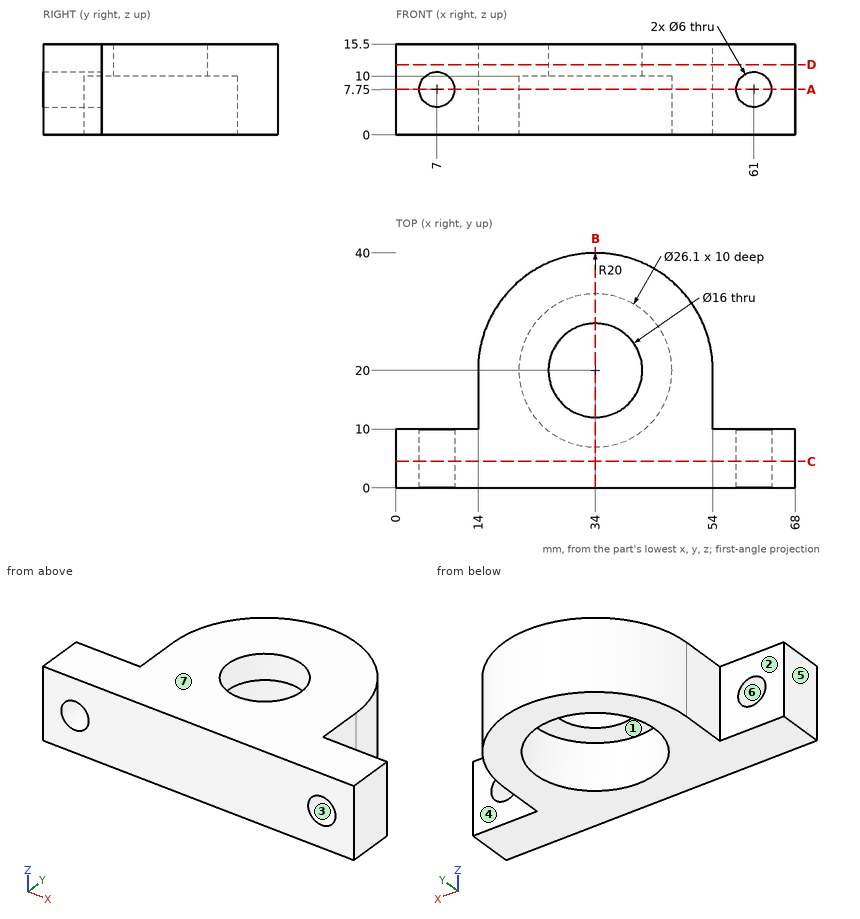
Geometry check sheet. Reference: drawing and pictorial views, mm from the part's lowest x, y, z. A direction names the side the tool comes from. Round coordinates to 2 decimals unless told otherwise and drop trailing zeros. Order: outer loops, then holes, each group sorted by start corner. A loop starts at its lowest first (then second) coordinate and runs counter-clockwise, first axis right, second up. Notation, with made-up numbers: M 46.5,68.5 L 71.5,68.5 A25 cw 71.5,106.5 Z; hole C -33.5,60.5 d2. An arc over 180 degrees is marked long. One line per item, written item: value. Start each with the question number.
1. Release check for a two-part mould opening along Z. For the marked faces 5, 6 and 7 record: released by +Z, released by -Z, zero draft, split by the parting line, or undercut.
2. Section check C-C on y = 4.5. Enter the section's corners in (x, z).
3. Section check A-A on z = 7.75. Enter the section's corners in (x, y), and give its area (3 significant figures).
4. Scan lines: line 1 along X through (y, z) = (5, 7.75); line 2 along Y through (x, z) = (34, 4.25); line 3 along Z through (x, y) = (61, 3.5). Record each from-to range of solid material in increasing order.
5. Section check B-B on x = 34. Enter the section's corners in (y, z), and give its area (3 significant figures).
6. Section check D-D on z = 12. Enter the section's corners in (x, y).
7. Access from +Z, -Z, +X, -X, +Y, -Y to the whole of each face (thin tool, end or side, straight path). Record for the marked faces 1, 2, 3 and 4.
8. Gauge pin test, flat ends, axial feed: P1, Ø1.5, axis at x = 34, z = 6, coming from the +Y side; P2, Ø2, axis at x = 8, z = 13, coming from the +Y side; P3, Ø3, axis at y = 25.5, z = 2, coming from the -X side; P4, Ø13, axis at x = 34, y = 20, coming from the -Z side. Record the tip position at first contact, or that the pin passes through.
Results found:
1. face 5: zero draft
1. face 6: undercut
1. face 7: released by +Z
2. outline: M 0,0 L 68,0 L 68,15.5 L 0,15.5 Z; hole C 7,7.75 d6; hole C 61,7.75 d6
3. outline: M 0,0 L 4,0 L 4,10 L 0,10 Z; M 10,0 L 58,0 L 58,10 L 54,10 L 54,20 A20 ccw 14,20 L 14,10 L 10,10 Z; M 64,0 L 68,0 L 68,10 L 64,10 Z; hole C 34,20 d26.1
3. area: 1,050 mm^2
4. line 1: 0 to 4, 10 to 58, 64 to 68
4. line 2: 0 to 6.95, 33.05 to 40
4. line 3: 0 to 4.75, 10.75 to 15.5
5. outline: M 0,0 L 6.95,0 L 6.95,10 L 12,10 L 12,15.5 L 0,15.5 Z; M 28,10 L 33.05,10 L 33.05,0 L 40,0 L 40,15.5 L 28,15.5 Z
5. area: 271 mm^2
6. outline: M 0,0 L 68,0 L 68,10 L 54,10 L 54,20 A20 ccw 14,20 L 14,10 L 0,10 Z; hole C 34,20 d16
7. face 1: -Z
7. face 2: +Z, -Z, -X, +Y
7. face 3: +Y, -Y
7. face 4: +Z, -Z, +X, +Y
8. P1: y = 40
8. P2: y = 10
8. P3: x = 14.4
8. P4: through
